Source: three-view drawing plus pictorial views. Frame: mm from the lowest corner of the part. Give positions to 0.01 mm unless a question says otherwise; leave off trailing zeros. Loops run counter-clockwise (first coordinate to the right, second up) from the corner with the lowest first, then second, coordinate; pieces in that order, holes last. Notation, with made-up numbers: (-4, 64.25) - (17, 64.25) arc R5 ccw to (17, 73.25) - close; hole circle Ø4 at (-11.75, 38.25). An arc over 180 degrees is marked (long way). Put each result on its own line as item: value.
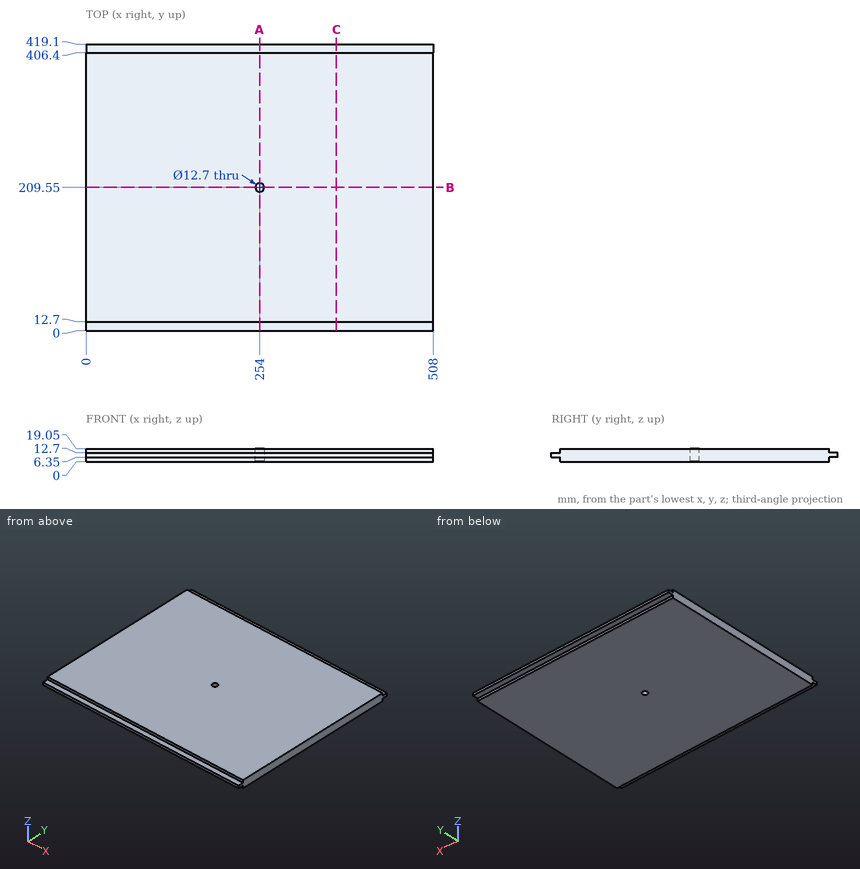
1) Section query A-A, the plane x = 254. Output: boundary loops of the cut face in (y, z).
Check result:
outline: (0, 6.35) - (12.7, 6.35) - (12.7, 0) - (203.2, 0) - (203.2, 19.05) - (12.7, 19.05) - (12.7, 12.7) - (0, 12.7) - close; (215.9, 0) - (406.4, 0) - (406.4, 6.35) - (419.1, 6.35) - (419.1, 12.7) - (406.4, 12.7) - (406.4, 19.05) - (215.9, 19.05) - close
2) Section query B-B, the plane y = 209.55. Output: boundary loops of the cut face in (x, z).
Check result:
outline: (0, 0) - (247.65, 0) - (247.65, 19.05) - (0, 19.05) - close; (260.35, 0) - (508, 0) - (508, 19.05) - (260.35, 19.05) - close
3) Material intervals for line 1 along Y through (x, z) = (254, 13.5); line 2 along Y through (x, z) = (254, 8.5); line 3 along Y through (x, z) = (25.5, 14.5), sorted ascending. Write a range as [from, to].
Check result:
line 1: [12.7, 203.2], [215.9, 406.4]
line 2: [0, 203.2], [215.9, 419.1]
line 3: [12.7, 406.4]
4) Section query C-C, the plane x = 366. Output: boundary loops of the cut face in (y, z), plus the area to 3 significant figures.
Check result:
outline: (0, 6.35) - (12.7, 6.35) - (12.7, 0) - (406.4, 0) - (406.4, 6.35) - (419.1, 6.35) - (419.1, 12.7) - (406.4, 12.7) - (406.4, 19.05) - (12.7, 19.05) - (12.7, 12.7) - (0, 12.7) - close
area: 7,660 mm²
5) Pin query (flat end, axial travel): P1, Ø6.5, axis at x = 167, y = 410, coming from the +Z side; P2, Ø6.5, axis at x = 352, y = 415.5, coming from the -Z side. Return the tip coordinate at first contact, or that it passes through.
Check result:
P1: z = 12.7
P2: z = 6.35
